Build history of the part. All positions in model axes, mm. Face numbers are marked on the shaded views. A direction names the side the tool comes from. Round coordinates to 2 decimals unless told otherwise and drop trailing zeros. Write each loop counter-clockwise with the first axis right and the second up, starting at its lowest first coordinate (ties: lowest second). Pieces come first, ordered by that corner, then holes.
from build123d import *

# Parameters (mm, degrees)
SKETCH2_W           = 970
SKETCH2_H           = 425
SKETCH2_W_2         = 966.825
SKETCH2_H_2         = 421.825
BOSS_EXTRUDE1_DEPTH = 420
BOSS_EXTRUDE2_START = 420
SKETCH3_W           = 970
SKETCH3_H           = 425
BOSS_EXTRUDE2_DEPTH = 1.5875
FILLET2_R           = 5


with BuildPart() as part:
    # Sketch2 → Boss-Extrude1 (new body)
    with BuildSketch(Plane(origin=(0, 0, 0), x_dir=(1, 0, 0), z_dir=(0, 1, 0))):
        Rectangle(SKETCH2_W, SKETCH2_H)
        Rectangle(SKETCH2_W_2, SKETCH2_H_2, mode=Mode.SUBTRACT)
    extrude(amount=BOSS_EXTRUDE1_DEPTH)

    # Sketch3 → Boss-Extrude2 (add)
    with BuildSketch(Plane(origin=(0, 0, 0), x_dir=(1, 0, 0), z_dir=(0, 1, 0)).offset(BOSS_EXTRUDE2_START)):
        Rectangle(SKETCH3_W, SKETCH3_H)
    extrude(amount=-BOSS_EXTRUDE2_DEPTH)

    # Fillet2
    fillet2_edges = [part.edges().sort_by_distance(p)[0] for p in [
        (-485, 420, 0),
        (0, 420, 212.5),
        (485, 420, 0),
        (485, 210, 212.5),
        (-485, 210, 212.5),
        (-485, 210, -212.5),
        (485, 210, -212.5),
        (0, 420, -212.5),
    ]]
    fillet(fillet2_edges, radius=FILLET2_R)


solid = part.part
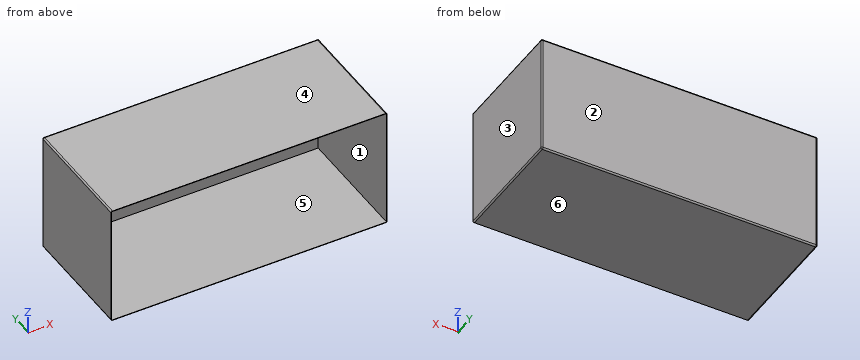
1) Slice it at A-A (x = 247). Write the cut outline in (y, z), plus the area to 3 significant figures.
Results:
outline: (0, -212.5) - (415, -212.5) arc R5 ccw to (420, -207.5) - (420, 207.5) arc R5 ccw to (415, 212.5) - (0, 212.5) - (0, 210.91) - (418.41, 210.91) - (418.41, -210.91) - (0, -210.91) - close
area: 1,990 mm2
2) Mould opens along Z. For the marked faces 3, 4, 5 and 6 say: released by +Z, released by -Z, zero draft, split by the parting line, or undercut.
Results:
face 3: zero draft
face 4: released by +Z
face 5: undercut
face 6: released by -Z
3) Slice it at B-B (z = -150.5). Write the cut outline in (x, y).
Results:
outline: (-485, 0) - (-483.41, 0) - (-483.41, 418.41) - (483.41, 418.41) - (483.41, 0) - (485, 0) - (485, 415) arc R5 ccw to (480, 420) - (-480, 420) arc R5 ccw to (-485, 415) - close
4) Which spindle directions (+Z, -Z, +X, -X, +Y, -Y) get a long thin tool onto all of the face, cutting with end or side? Do the marked faces 1 and 2. Say none if no direction does.
Results:
face 1: -Y
face 2: +Z, -Z, +X, -X, +Y
5) Slice it at C-C (y = 237). Write the cut outline in (x, z).
Results:
outline: (-485, -207.5) arc R5 ccw to (-480, -212.5) - (480, -212.5) arc R5 ccw to (485, -207.5) - (485, 207.5) arc R5 ccw to (480, 212.5) - (-480, 212.5) arc R5 ccw to (-485, 207.5) - close; hole (-483.41, -210.91) - (483.41, -210.91) - (483.41, 210.91) - (-483.41, 210.91) - close
6) Wall check: L1, parallel to Z at x = 118, y = 191; L2, parallel to X at y = 284.5, z = 11.5; L3, parallel to Y at x = -379.5, z = -134. Give the ranges that are in metal, low to high.
Results:
L1: z = -212.5 to -210.91, 210.91 to 212.5
L2: x = -485 to -483.41, 483.41 to 485
L3: y = 418.41 to 420
